```python
from build123d import *

# Parameters (mm, degrees)
SKETCH2_W               = 590.8
SKETCH2_H               = 600
BASE_FLANGE1_DEPTH      = 1.016
EDGE_FLANGE1_DEPTH      = 600
EDGE_FLANGE1_BEND_DEPTH = 600
CUT_EXTRUDE1_DEPTH      = 845.862743377
CUT_EXTRUDE1_DEPTH_BACK = 845.862743377
SKETCH31_W              = 55.3
SKETCH31_H              = 22.226


# Sheet-metal steps are written as plain solids
with BuildPart() as part:
    # Sketch2 → Base-Flange1 (new body)
    with BuildSketch(Plane(origin=(0, 0, 0), x_dir=(1, 0, 0), z_dir=(0, 1, 0))):
        with Locations((295.4, 300)):
            Rectangle(SKETCH2_W, SKETCH2_H)
    extrude(amount=-BASE_FLANGE1_DEPTH)

    # Edge-Flange1 section (across the edge) → Edge-Flange1 (add)
    with BuildSketch(Plane(origin=(-0.7366, 0, -600), x_dir=(1, 0, 0), z_dir=(0, 0, 1))):
        with BuildLine():
            Line((-1.016, 0.7366), (-1.016, 24.38))
            Line((-1.016, 24.38), (0, 24.38))
            Line((0, 24.38), (0, 0.7366))
            ThreePointArc((0, 0.7366), (0.215745145, 0.215745145), (0.7366, 0))
            Line((0.7366, 0), (0.7366, -1.016))
            ThreePointArc((0.7366, -1.016), (-0.502675345, -0.502675345), (-1.016, 0.7366))
        make_face()
    extrude(amount=EDGE_FLANGE1_DEPTH)

    # Edge-Flange1 section 2 (across the edge) → Edge-Flange1 bend (add)
    with BuildSketch(Plane(origin=(591.5366, 0, 0), x_dir=(-1, 0, 0), z_dir=(0, 0, -1))):
        with BuildLine():
            Line((-1.016, 0.7366), (-1.016, 24.38))
            Line((-1.016, 24.38), (0, 24.38))
            Line((0, 24.38), (0, 0.7366))
            ThreePointArc((0, 0.7366), (0.215745145, 0.215745145), (0.7366, 0))
            Line((0.7366, 0), (0.7366, -1.016))
            ThreePointArc((0.7366, -1.016), (-0.502675345, -0.502675345), (-1.016, 0.7366))
        make_face()
    extrude(amount=EDGE_FLANGE1_BEND_DEPTH)

    # Sketch31 → Cut-Extrude1 (cut, two sides: drawn at the far end of the back side and taken through both)
    with BuildSketch(Plane.ZY.offset(1.7526).offset(-CUT_EXTRUDE1_DEPTH_BACK)):
        with Locations((-350, 13.267)):
            Rectangle(SKETCH31_W, SKETCH31_H)
    extrude(amount=CUT_EXTRUDE1_DEPTH + CUT_EXTRUDE1_DEPTH_BACK, mode=Mode.SUBTRACT)


solid = part.part
```
Design review of the part built by this model. Coordinates are the model's own, in mm. A direction names the side the tool comes from. Coordinates: 2 decimals unless noted, no trailing zeros. Order: outer loops, then holes, each group sorted by start corner. A loop starts at its lowest first (then second) coordinate and runs counter-clockwise, first axis right, second up.
1) Clearance check with flat-ended pins moving along their axes: pin 1 (0.8 mm diameter, centred on x = -1, z = -363.5, fed in from +Y); pin 2 (2 mm diameter, centred on x = 124, z = -73, fed in from +Y). State where each tip first meets the part, or that it passes through.
2) Take a section at B-B, the plane z = -106.5. Give the boundary of the cut face in (x, y).
3) Take a section at C-C, the plane x = 463.5. Give the boundary of the cut face in (y, z).
4) For faces 1 (the flat face through (-0.737, 13, -304)), 2 (the flat face through (-1.753, 12, -304)), list the 3-axis set-ups (+Z, -Z, +X, -X, +Y, -Y) from which the entire face can be reached by the end or side of a thin tool; tool diameter is ignored.
5) Take a section at A-A, the plane y = 12.5. Give the boundary of the cut face in (x, z).
6) Mouldability with a two-part tool opening along Z and no side actions: class faces 3 (the flat face through (592.553, 12, -296)), 4 (the flat face through (294, -0.5, -600)), 5 (the flat face through (294, -0.5, 0)) as +Z half, -Z half, draft (parallel to the pull), parting line (faces both ways), or undercut.
7) Wall thickness on line 1 along X through (y, z) = (8.75, -427); line 2 along Y through (x, z) = (551, -38.5): over which ranges is each line inside the solid? List them lowest first.
Returned:
1. pin 1: stops at y = 2.15
1. pin 2: stops at y = 0
2. outline: (-1.75, 0.74) arc R1.75 ccw to (0, -1.02) - (590.8, -1.02) arc R1.75 ccw to (592.55, 0.74) - (592.55, 24.38) - (591.54, 24.38) - (591.54, 0.74) arc R0.74 cw to (590.8, 0) - (0, 0) arc R0.74 cw to (-0.74, 0.74) - (-0.74, 24.38) - (-1.75, 24.38) - close
3. outline: (-1.02, -600) - (0, -600) - (0, 0) - (-1.02, 0) - close
4. face 1: +Z, -Z, +Y
4. face 2: +Z, -Z, -X, +Y, -Y
5. outline: (-1.75, -600) - (-0.74, -600) - (-0.74, -377.65) - (-1.75, -377.65) - close; (-1.75, -322.35) - (-0.74, -322.35) - (-0.74, 0) - (-1.75, 0) - close; (591.54, -600) - (592.55, -600) - (592.55, -377.65) - (591.54, -377.65) - close; (591.54, -322.35) - (592.55, -322.35) - (592.55, 0) - (591.54, 0) - close
6. face 3: draft
6. face 4: -Z half
6. face 5: +Z half
7. line 1: x = -1.75 to -0.74, 591.54 to 592.55
7. line 2: y = -1.02 to 0
